Here's how the part is built. I have some questions about the finished solid (model axes, mm). Round coordinates to 2 decimals unless told otherwise and drop trailing zeros. Write each loop counter-clockwise with the first axis right and the second up, starting at its lowest first coordinate (ties: lowest second). Pieces come first, ordered by that corner, then holes. Notation, with made-up numbers: (22.25, 67) -> (77.25, 67) arc R35 cw to (77.25, 105) -> close; hole circle Ø3 at (79, 32.5). An arc over 180 degrees is marked (long way). Answer in a Markdown table with one row per item.
from build123d import *

# Parameters (mm, degrees)
SKETCH1_R           = 4.7625
BOSS_EXTRUDE1_DEPTH = 9.525


with BuildPart() as part:
    # Sketch1 → Boss-Extrude1 (new body)
    with BuildSketch(Plane(origin=(0, 0, 0), x_dir=(0, 0, -1), z_dir=(1, 0, 0))):
        Polygon((0, 8.248891971), (-7.14375, 4.124445986), (-7.14375, -4.124445986), (0, -8.248891971), (7.14375, -4.124445986), (7.14375, 4.124445986), align=None)
        Circle(SKETCH1_R, mode=Mode.SUBTRACT)
    extrude(amount=BOSS_EXTRUDE1_DEPTH)

    # Sketch2 → Cut-Revolve1 (revolve, cut)
    with BuildSketch(Plane.XY):
        Polygon((0, 7.14375), (0.402238782, 8.248891971), (0, 8.248891971), align=None)
        Polygon((0, 4.7625), (0.254, 4.7625), (0, 5.0165), align=None)
        Polygon((9.525, 5.0165), (9.525, 4.7625), (9.271, 4.7625), align=None)
        Polygon((9.525, 8.248891971), (9.525, 7.14375), (9.122761218, 8.248891971), align=None)
    revolve(axis=Axis((0, 0, 0), (1, 0, 0)), mode=Mode.SUBTRACT)


solid = part.part
1) For pin 1 (3 mm diameter, centred on x = 8, z = -2, fed in from +Y); pin 2 (4 mm diameter, centred on y = 4.5, z = -0.5, fed in from -X); pin 3 (8.5 mm diameter, centred on y = 0, z = 0, fed in from +X), each with a flat end and sliding along its axis, tell me the tip position at first contact or that it passes through.
Response:
| item | result |
|---|---|
| pin 1 | stops at y = 7.96 |
| pin 2 | stops at x = 0 |
| pin 3 | passes through |
2) I need wall thicknesses on line 1 (Z direction, x = 5.75, y = -3); line 2 (Y direction, x = 9, z = -2.5); line 3 (Y direction, x = 2, z = 0.25). Which ranges of each line are inside material? Lowest first, please. Write a range as [from, to].
Response:
| item | result |
|---|---|
| line 1 | z = [-7.14, -3.7], [3.7, 7.14] |
| line 2 | y = [-6.81, -4.05], [4.05, 6.81] |
| line 3 | y = [-8.1, -4.76], [4.76, 8.1] |
3) I want a section at A-A, the plane x = 8.5. List the corners of the cut face in (y, z) for me (1 decimal), and give its area (3 significant figures).
Response:
| item | result |
|---|---|
| outline | (-8.2, 0) -> (-4.1, -7.1) -> (4.1, -7.1) -> (8.2, 0) -> (4.1, 7.1) -> (-4.1, 7.1) -> close; hole circle Ø9.5 at (0, 0) |
| area | 106 mm^2 |
4) We'd pull the mould along Y, two halves only. Please class faces 1 (the face through (4.7, -1.82, -4.4)), 2 (the face through (9.427, -3.722, -6.41)), 3 (the face through (5, 0, -7.144)), 4 (the face through (9.43, 7.41, -0.02)): +Y half, -Y half, draft (parallel to the pull), parting line (faces both ways), or undercut.
Response:
| item | result |
|---|---|
| face 1 | undercut |
| face 2 | -Y half |
| face 3 | draft |
| face 4 | +Y half |
